The model under review builds one solid part; all positions refer to its coordinate system, in mm. A direction names the side the tool comes from. Round coordinates to 2 decimals unless told otherwise and drop trailing zeros. Order: outer loops, then holes, each group sorted by start corner. A loop starts at its lowest first (then second) coordinate and runs counter-clockwise, first axis right, second up. Notation, with made-up numbers: M 2.5,35.25 L 58.5,35.25 A23 ccw 58.5,49.25 Z; hole C -2,-27 d9. An arc over 180 degrees is marked long. Answer as a JSON object with one key per item and string values. Group by question number.
1) Consider section C-C, the plane z = -6. Write out the cut boundary in (x, y).
2) Consider section B-B, the plane y = 32.5. Write out the cut boundary in (x, z), then the cut area to 3 significant figures.
3) Consider section D-D, the plane z = 29. Write out the cut boundary in (x, y), then the cut area to 3 significant figures.
4) Consider section A-A, the plane x = -34.5. Write out the cut boundary in (y, z), then the cut area to 3 significant figures.
5) Insertion check: pin 1 Ø0.9 at (y, z) = (80, -23) entering from +X; pin 2 Ø5.5 at (x, y) = (-81.5, 45) entering from +Z; pin 3 Ø3.5 at (y, z) = (79, -28.5) entering from -X. Each pin has a flat end and moves straight along its axis. Give the tip position at first contact, or say it passes through.
6) To check wall thickness, follow line 1 (X direction, y = 49, z = -7.5); line 2 (Z direction, x = 0, y = 2.25); line 3 (Z direction, x = 81, y = 13). State the ranges of each line that lie inside material, in increasing order.
7) The part is to be moulded in two halves that separate along Y. For faces 1 (the flat face through (-1, 0, 0)), 2 (the flat face through (-77, 28, 15.368)), 3 (the flat face through (-83, 3, 0)), 4 (the flat face through (-77, 40, 0)), say which applies: +Y half, -Y half, draft (parallel to the pull), parting line (faces both ways), or undercut.
8) For faces 5 (the cylindrical face through (0, 1, 20)), 6 (the flat face through (90, 40, 0)), 7 (the flat face through (88, 40, 0)), 8 (the cylindrical face through (0, 1, -20)), 9 (the flat face through (75, 40, 0)), list the 3-axis set-ups (+Z, -Z, +X, -X, +Y, -Y) from which the entire face can be reached by the end or side of a thin tool; tool diameter is ignored.
```python
from build123d import *

# Parameters (mm, degrees)
F0_R     = 1
F1_DEPTH = 3
F2_DEPTH = 81
F4_W     = 73
F4_H     = 15.3680173474
F4_W_2   = 34
F4_H_2   = 18.6319826526
F5_DEPTH = 3
F6_DEPTH = 3


with BuildPart() as f1:
    # F0 (on Front) → F1 (new body)
    with BuildSketch(Plane.XZ):
        with BuildLine():
            Line((-75, -15.3680173474), (-12.7993766571, -15.3680173474))
            ThreePointArc((-12.7993766571, -15.3680173474), (-18.1105981837, -8.4856486746), (-20, 0))
            Line((-20, 0), (-69, 0))
            Line((-69, 0), (-75, 0))
            Line((-75, 0), (-75, -15.3680173474))
        make_face()
        with BuildLine():
            ThreePointArc((-20, 0), (-18.1105981837, 8.4856486746), (-12.7993766571, 15.3680173474))
            Line((-12.7993766571, 15.3680173474), (-75, 15.3680173474))
            Line((-75, 15.3680173474), (-75, 0))
            Line((-75, 0), (-69, 0))
            Line((-69, 0), (-20, 0))
        make_face()
        with BuildLine():
            ThreePointArc((12.7993766571, 15.3680173474), (18.1105981837, 8.4856486746), (20, 0))
            Line((20, 0), (69, 0))
            Line((69, 0), (75, 0))
            Line((75, 0), (75, 15.3680173474))
            Line((75, 15.3680173474), (12.7993766571, 15.3680173474))
        make_face()
        with BuildLine():
            Line((69, 0), (20, 0))
            ThreePointArc((20, 0), (18.1105981837, -8.4856486746), (12.7993766571, -15.3680173474))
            Line((12.7993766571, -15.3680173474), (75, -15.3680173474))
            Line((75, -15.3680173474), (75, 0))
            Line((75, 0), (69, 0))
        make_face()
        with BuildLine():
            Line((18, 0), (20, 0))
            ThreePointArc((20, 0), (18.1105981837, 8.4856486746), (12.7993766571, 15.3680173474))
            ThreePointArc((12.7993766571, 15.3680173474), (0, 20), (-12.7993766571, 15.3680173474))
            ThreePointArc((-12.7993766571, 15.3680173474), (-18.1105981837, 8.4856486746), (-20, 0))
            Line((-20, 0), (-18, 0))
            ThreePointArc((-18, 0), (-17, 1), (-16, 0))
            Line((-16, 0), (0, 0))
            Line((0, 0), (16, 0))
            ThreePointArc((16, 0), (17, 1), (18, 0))
        make_face()
        with Locations((0, 17)):
            Circle(F0_R, mode=Mode.SUBTRACT)
        with BuildLine():
            ThreePointArc((12.7993766571, -15.3680173474), (18.1105981837, -8.4856486746), (20, 0))
            Line((20, 0), (18, 0))
            ThreePointArc((18, 0), (17, -1), (16, 0))
            Line((16, 0), (0, 0))
            Line((0, 0), (-16, 0))
            ThreePointArc((-16, 0), (-17, -1), (-18, 0))
            Line((-18, 0), (-20, 0))
            ThreePointArc((-20, 0), (-18.1105981837, -8.4856486746), (-12.7993766571, -15.3680173474))
            ThreePointArc((-12.7993766571, -15.3680173474), (0, -20), (12.7993766571, -15.3680173474))
        make_face()
        with Locations((0, -17)):
            Circle(F0_R, mode=Mode.SUBTRACT)
    extrude(amount=-F1_DEPTH)

    # F0 (on Front) → F2 (join)
    with BuildSketch(Plane.XZ):
        Polygon((90, 15.3680173474), (75, 15.3680173474), (75, 0), (75, -15.3680173474), (90, -15.3680173474), align=None)
        Polygon((77, 0), (77, 13.3680173474), (88, 13.3680173474), (88, -13.3680173474), (77, -13.3680173474), align=None, mode=Mode.SUBTRACT)
        Polygon((-75, 0), (-75, 15.3680173474), (-90, 15.3680173474), (-90, -15.3680173474), (-75, -15.3680173474), align=None)
        Polygon((-88, -13.3680173474), (-88, 13.3680173474), (-77, 13.3680173474), (-77, 0), (-77, -13.3680173474), align=None, mode=Mode.SUBTRACT)
    extrude(amount=-F2_DEPTH)

    # F4 (on offset) → F5 (join)
    with BuildSketch(Plane.XZ.offset(-81)):
        with Locations((53.5, 7.6840086737)):
            Rectangle(F4_W, F4_H)
        with Locations((53.5, -7.6840086737)):
            Rectangle(F4_W, F4_H)
        Polygon((-17, 0), (0, 0), (17, 0), (17, 15.3680173474), (-17, 15.3680173474), align=None)
        with Locations((0, 24.6840086737)):
            Rectangle(F4_W_2, F4_H_2)
        Polygon((17, 0), (0, 0), (-17, 0), (-17, -15.3680173474), (17, -15.3680173474), align=None)
        with Locations((0, -24.6840086737)):
            Rectangle(F4_W_2, F4_H_2)
        with Locations((-53.5, -7.6840086737)):
            Rectangle(F4_W, F4_H)
        with Locations((-53.5, 7.6840086737)):
            Rectangle(F4_W, F4_H)
    extrude(amount=F5_DEPTH)

    # F0 (on Front) → F6 (join)
    with BuildSketch(Plane.XZ):
        Polygon((88, 13.3680173474), (77, 13.3680173474), (77, 0), (77, -13.3680173474), (88, -13.3680173474), align=None)
        Polygon((-77, 13.3680173474), (-88, 13.3680173474), (-88, -13.3680173474), (-77, -13.3680173474), (-77, 0), align=None)
    extrude(amount=-F6_DEPTH)


solid = f1.part
```
Results list:
{
 "1": {"outline": "M -90,0 L 90,0 L 90,81 L -90,81 Z; hole M -88,3 L -77,3 L -77,78 L -88,78 Z; hole M -75,3 L 75,3 L 75,78 L -75,78 Z; hole M 77,3 L 88,3 L 88,78 L 77,78 Z"},
 "2": {"outline": "M -90,-15.37 L -75,-15.37 L -75,15.37 L -90,15.37 Z; M 75,-15.37 L 90,-15.37 L 90,15.37 L 75,15.37 Z; hole M -88,-13.37 L -77,-13.37 L -77,13.37 L -88,13.37 Z; hole M 77,-13.37 L 88,-13.37 L 88,13.37 L 77,13.37 Z", "area": "334 mm^2"},
 "3": {"outline": "M -17,78 L 17,78 L 17,81 L -17,81 Z", "area": "102 mm^2"},
 "4": {"outline": "M 0,-15.37 L 3,-15.37 L 3,15.37 L 0,15.37 Z; M 78,-15.37 L 81,-15.37 L 81,15.37 L 78,15.37 Z", "area": "184 mm^2"},
 "5": {"pin 1": "x = 17", "pin 2": "z = 15.37", "pin 3": "x = -17"},
 "6": {"line 1": "-90 to -88, -77 to -75, 75 to 77, 88 to 90", "line 2": "-20 to -18, -16 to 16, 18 to 20", "line 3": "-15.37 to -13.37, 13.37 to 15.37"},
 "7": {"face 1": "-Y half", "face 2": "draft", "face 3": "undercut", "face 4": "undercut"},
 "8": {"face 5": "+Z, -Y", "face 6": "+Z, -Z, +X, +Y, -Y", "face 7": "none", "face 8": "-Z, -Y", "face 9": "+Z, -Z"}
}
